Here's how the part is built. I have some questions about the finished solid (model axes, mm). A direction names the side the tool comes from. Coordinates: 2 decimals unless noted, no trailing zeros. Write each loop counter-clockwise with the first axis right and the second up, starting at its lowest first coordinate (ties: lowest second). Pieces come first, ordered by that corner, then holes.
Item 1: I want a section at C-C (x = 0). Please give me the cut outline in (y, z).
Item 2: I want a section at D-D (y = 20.95). Please give me the cut outline in (x, z).
Item 3: If we mould it in two halves opening along Z, with no side actions, what happens to faces 1 (the face through (-1, 21, -115.8)), 2 (the face through (-1, 11, 115.8)), 3 (the face through (-40.735, 0.986, 0.976)), 4 (the face through (-1, 0, -2))? For each: pulls with the +Z half, pulls with the -Z half, needs draft (parallel to the pull), parting line crosses it, or undercut.
Item 4: For faces 5 (the face through (-1, 22, -113.8)), 6 (the face through (0.7, 16, 120.7)), 7 (the face through (0, 21, 125.8)), which set-ups out of +Z, -Z, +X, -X, +Y, -Y let a thin tool reach every point of the face, with its end or its side?
Item 5: I'm going to push flat-ended pins straight in: P1, Ø1.6, axis at y = 3, z = -114.5, coming from the +X side; P2, Ø1, axis at x = 94.5, z = -114.5, coming from the -Y side; P3, Ø8, axis at x = -65, z = 57.5, coming from the +Y side; P4, Ø6, axis at x = -67.5, y = 29.5, coming from the +Z side. Where does each tip first touch, or does it pass through?
Item 6: I want a section at A-A (y = 38). Please give me the cut outline in (x, z).
Item 7: I want a section at B-B (z = 0). Please give me the cut outline in (x, y).
Item 8: Please list where these lines run through material, in increasing order: line 1 (X direction, y = 1.15, z = 0); line 2 (Z direction, x = -21, y = 39); line 3 (Y direction, x = 65, z = 16.5).
from build123d import *

# Parameters (mm, degrees)
SKETCH_2_W         = 191.4
SKETCH_2_H         = 231.6
EXTRUDE_1_DEPTH    = 2
SKETCH_3_W         = 185
SKETCH_3_H         = 2
EXTRUDE_2_DEPTH    = 2.5
SKETCH_4_W         = 191.4
SKETCH_4_H         = 2
EXTRUDE_3_DEPTH    = 37.4
SKETCH_7_R         = 5
EXTRUDE_5_DEPTH    = 10
SKETCH1_R          = 7.5
CUT_EXTRUDE1_DEPTH = 10


with BuildPart() as part:
    # 草图2 → 凸台-拉伸1 (new body)
    with BuildSketch(Plane(origin=(0, 0, 0), x_dir=(1, 0, 0), z_dir=(0, 1, 0))):
        Rectangle(SKETCH_2_W, SKETCH_2_H)
    extrude(amount=EXTRUDE_1_DEPTH)

    # 草图3 → 凸台-拉伸2 (add)
    with BuildSketch(Plane(origin=(0, 2, 0), x_dir=(1, 0, 0), z_dir=(0, 1, 0))):
        with Locations((0, 114.8)):
            Rectangle(SKETCH_3_W, SKETCH_3_H)
        with Locations((0, -114.8)):
            Rectangle(SKETCH_3_W, SKETCH_3_H)
    extrude(amount=EXTRUDE_2_DEPTH)

    # 草图4 → 凸台-拉伸3 (add)
    with BuildSketch(Plane(origin=(0, 4.5, 0), x_dir=(1, 0, 0), z_dir=(0, 1, 0))):
        with Locations((0, 114.8)):
            Rectangle(SKETCH_4_W, SKETCH_4_H)
        with Locations((0, -114.8)):
            Rectangle(SKETCH_4_W, SKETCH_4_H)
    extrude(amount=EXTRUDE_3_DEPTH)

    # 草图7 → 凸台-拉伸5 (add)
    with BuildSketch(Plane.XY.offset(115.8)):
        with Locations(Location((0, 20.95, 0), (0, 0, 180))):
            Circle(SKETCH_7_R)
    extrude(amount=EXTRUDE_5_DEPTH)

    # Sketch1 → Cut-Extrude1 (cut)
    with BuildSketch(Plane.XZ):
        with Locations(Location((-48.170733531, 0, 0), (0, 0, 270))):
            Circle(SKETCH1_R)
    extrude(amount=-CUT_EXTRUDE1_DEPTH, mode=Mode.SUBTRACT)


solid = part.part
Answer:
1. outline: (0, -115.8) - (41.9, -115.8) - (41.9, -113.8) - (2, -113.8) - (2, 113.8) - (41.9, 113.8) - (41.9, 115.8) - (25.95, 115.8) - (25.95, 125.8) - (15.95, 125.8) - (15.95, 115.8) - (0, 115.8) - close
2. outline: (-95.7, -115.8) - (95.7, -115.8) - (95.7, -113.8) - (-95.7, -113.8) - close; (-95.7, 113.8) - (95.7, 113.8) - (95.7, 115.8) - (5, 115.8) - (5, 125.8) - (-5, 125.8) - (-5, 115.8) - (-95.7, 115.8) - close
3. face 1: pulls with the -Z half
3. face 2: pulls with the +Z half
3. face 3: undercut
3. face 4: needs draft
4. face 5: +X, -X, +Y
4. face 6: +Z
4. face 7: +Z, +X, -X, +Y, -Y
5. P1: stops at x = 92.5
5. P2: stops at y = 0
5. P3: stops at y = 2
5. P4: stops at z = 115.8
6. outline: (-95.7, -115.8) - (95.7, -115.8) - (95.7, -113.8) - (-95.7, -113.8) - close; (-95.7, 113.8) - (95.7, 113.8) - (95.7, 115.8) - (-95.7, 115.8) - close
7. outline: (-95.7, 0) - (-55.67, 0) - (-55.67, 2) - (-95.7, 2) - close; (-40.67, 0) - (95.7, 0) - (95.7, 2) - (-40.67, 2) - close
8. line 1: x = -95.7 to -55.67, -40.67 to 95.7
8. line 2: z = -115.8 to -113.8, 113.8 to 115.8
8. line 3: y = 0 to 2
